Here's how the part is built. I have some questions about the finished solid (model axes, mm). A direction names the side the tool comes from. Give positions to 0.01 mm unless a question says otherwise; leave off trailing zeros. Loops run counter-clockwise (first coordinate to the right, second up) from the corner with the lowest first, then second, coordinate; pieces in that order, holes last. Notation, with made-up numbers: (74.5, 27) - (127.5, 27) arc R25 cw to (127.5, 66) - close; hole circle Ø2 at (23, 78.5). An arc over 180 degrees is marked (long way). Return JSON: item names as keys, results as strings. Group by question number.
(1) If we section it at A-A (y = 5.5): Please give me the cut outline in (x, z).
(2) I need wall thicknesses on probe 1 along Y at (x, z) = (5.5, 1.5); probe 2 along Z at (x, y) = (10.25, 1). Which ranges of each line are inside material? Lowest first, please. Write a range as [from, to].
(3) If we mould it in two halves opening along Z, with no side actions, what happens to faces 3 (the cylindrical face through (10.43, 25.25, -45.85)), 4 (the flat face through (12.4, -43, 26))? For each: released by +Z, released by -Z, zero draft, split by the parting line, or undercut.
(4) On a 3-axis mill with a long thin cutter (end or side, diameter ignored), from which of +Z, -Z, +X, -X, +Y, -Y can I reach the whole of each face in a straight line? I mean faces 1 (the cylindrical face through (3.926, -26.945, -48.014)), 2 (the cylindrical face through (10.428, -27.087, -44.792)). Say none if no direction works.
(5) For P1, Ø4, axis at x = 7, y = -45, coming from the +Z side; P2, Ø3, axis at y = 0, z = -54, coming from the +X side; P3, Ø5, axis at x = 7.5, z = 3, coming from the +Y side, each with a flat end and sliding along its axis, tell me the tip position at first contact or that it passes through.
(6) If we section it at B-B (z = -4.5): Please give me the cut outline in (x, y).
```python
from build123d import *

# Parameters (mm, degrees)
SKETCH_1_W               = 9.9
SKETCH_1_H               = 7.8
SKETCH_1_W_2             = 2.5
SKETCH_1_H_2             = 9.8
HOLE_WIZARD_M3_1_D       = 2.5
PATTERN_CIRCULAR_1_COUNT = 12


with BuildPart() as part:
    # Sketch 1 → Revolve 1 (revolve)
    with BuildSketch(Plane.XY, mode=Mode.PRIVATE) as revolve_1_sk:
        with Locations((7.45, 53.9)):
            Rectangle(SKETCH_1_W, SKETCH_1_H)
        with Locations((1.25, 52.9)):
            Rectangle(SKETCH_1_W_2, SKETCH_1_H_2)
    revolve(revolve_1_sk.sketch.rotate(Axis((0, 0, 0), (1, 0, 0)), 90), axis=Axis((0, 0, 0), (1, 0, 0)))

    # Hole Wizard M3 _1 (through all)
    with Locations(Plane(origin=(12.4, 0, 0), x_dir=(0, 0, -1), z_dir=(1, 0, 0))):
        with Locations((0, 54)):
            hole_wizard_m3_1 = Hole(HOLE_WIZARD_M3_1_D / 2)

    # Sketch 9 → 4.0mm _1 (revolve, cut)
    with BuildSketch(Plane(origin=(12.4, 54, 0), x_dir=(0, 0, -1), z_dir=(0, 1, 0))):
        Polygon((0, 0), (0, 5.186699723), (1.975, 4), (1.975, 0), align=None)
    f_4_0mm_1 = revolve(axis=Axis((18.75, 54, 0), (-1, 0, 0)), mode=Mode.SUBTRACT)

    # Pattern Circular 1: Hole Wizard M3 _1, 4.0mm _1 ×12 about axis
    pattern_circular_1_axis = Axis((0, 0, 0), (1, 0, 0))
    add([hole_wizard_m3_1.rotate(pattern_circular_1_axis, i * 360 / PATTERN_CIRCULAR_1_COUNT) for i in range(1, PATTERN_CIRCULAR_1_COUNT)], mode=Mode.SUBTRACT)
    add([f_4_0mm_1.rotate(pattern_circular_1_axis, i * 360 / PATTERN_CIRCULAR_1_COUNT) for i in range(1, PATTERN_CIRCULAR_1_COUNT)], mode=Mode.SUBTRACT)


solid = part.part
```
Values:
{
 "1": {"outline": "(0, -57.54) - (12.4, -57.54) - (12.4, -49.7) - (2.5, -49.7) - (2.5, -47.68) - (0, -47.68) - close; (0, 47.68) - (2.5, 47.68) - (2.5, 49.7) - (12.4, 49.7) - (12.4, 57.54) - (0, 57.54) - close"},
 "2": {"probe 1": "[-57.78, -49.98], [49.98, 57.78]", "probe 2": "[-57.79, -55.7], [-52.3, -49.99], [49.99, 52.3], [55.7, 57.79]"},
 "3": {"face 3": "undercut", "face 4": "zero draft"},
 "4": {"face 1": "+X, -X", "face 2": "+X"},
 "5": {"P1": "z = 38.62", "P2": "x = 8.11", "P3": "y = 57.8"},
 "6": {"outline": "(0, -57.62) - (12.4, -57.62) - (12.4, -49.8) - (2.5, -49.8) - (2.5, -47.79) - (0, -47.79) - close; (0, 47.79) - (2.5, 47.79) - (2.5, 49.8) - (12.4, 49.8) - (12.4, 57.62) - (0, 57.62) - close"}
}
